Autodesk Inventor part; units mm, degrees
ref_plane "YZ Plane" through (0, 0, 0) normal (1, 0, 0) x (0, 1, 0)
ref_plane "XZ Plane" through (0, 0, 0) normal (0, 1, 0) x (-1, 0, 0)
ref_plane "XY Plane" through (0, 0, 0) normal (0, 0, 1) x (1, 0, 0)
sketch "Sketch1" plane through (0, 0, 0) normal (0, 1, 0) x (-1, 0, 0)
  circle A0 centre (0, 0) radius 4
  arc A1 (-5.0181, 4.8805) -> (5.0181, 4.8805) centre (0, 0) ccw
  arc A2 (9.6094, 20.8964) -> (-9.6094, 20.8964) centre (0, 0) ccw
  arc A3 (-5.0181, 4.8805) -> (-9.6094, 20.8964) centre (-11.9, 11.5737) ccw
  arc A4 (9.6094, 20.8964) -> (5.0181, 4.8805) centre (11.9, 11.5737) ccw
  line L0 (5.0181, 4.8805) -> (-5.0181, 4.8805)
  dimension "d0" = 8
  dimension "d1" = 14
  dimension "d2" = 46
  dimension "d15" = 9.6
  dimension "d17" = 4.6
extrude "Extrusion3" add sketch "Sketch1" along normal blind 1.5
properties part number "crusher_claw"
Model file for the job. Use its own axes, mm. Round coordinates to 2 decimals unless told otherwise and drop trailing zeros. Loops run counter-clockwise (first coordinate to the right, second up) from the corner with the lowest first, then second, coordinate; pieces in that order, holes last. Notation, with made-up numbers: M 73,-37.75 L 100,-37.75 A15 ccw 100,-28.75 Z; hole C 74,65 d11. An arc over 180 degrees is marked long. Put each result on its own line as item: value. Start each with the question number.
Item 1: Mould opens along Z. For faces 1 (the face through (0, 1, 23)), 2 (the face through (0, 0, 8)), 3 (the face through (-2.634, 0.74, 14.083)), 4 (the face through (2.71, 0.74, 14.35)) say: released by +Z, released by -Z, zero draft, split by the parting line, or undercut.
Item 2: Cut at C-C (x = -2.75). List the corners of the cut face in (y, z) (3 decimals), then the cut area to 3 significant figures.
Item 3: Cut at B-B (x = 6.5). List the corners of the cut face in (y, z), then the cut area to 3 significant figures.
Item 4: Cut at D-D (y = 0.25). List the corners of the cut face in (x, z).
Item 5: Drop a flat-ended pin along its axis: P1, Ø6, axis at x = -2, z = 14, coming from the -Y side. Give the stop position or say it passes through.
Item 6: Drill centre lines: line 1 along Z through (x, y) = (0, 0.95); line 2 along X through (y, z) = (1.4, -1.5); line 3 along X through (y, z) = (1.15, -2). Where is each one in solid material? Low to high.
Item 7: Cut at A-A (z = 0). List the corners of the cut face in (x, y), then the cut area to 3 significant figures.
Answer block:
1. face 1: released by +Z
1. face 2: zero draft
1. face 3: undercut
1. face 4: undercut
2. outline: M 0,-6.437 L 1.5,-6.437 L 1.5,-2.905 L 0,-2.905 Z; M 0,2.905 L 1.5,2.905 L 1.5,8.669 L 0,8.669 Z; M 0,14.478 L 1.5,14.478 L 1.5,22.835 L 0,22.835 Z
2. area: 26.5 mm2
3. outline: M 0,-2.6 L 1.5,-2.6 L 1.5,2.6 L 0,2.6 Z; M 0,19.51 L 1.5,19.51 L 1.5,22.06 L 0,22.06 Z
3. area: 11.6 mm2
4. outline: M -9.61,20.9 A9.6 cw -5.02,4.88 A7 ccw long 5.02,4.88 A9.6 cw 9.61,20.9 A23 ccw Z; hole C 0,0 d8
5. P1: y = 0
6. line 1: -7 to -4, 4 to 23
6. line 2: -6.84 to -3.71, 3.71 to 6.84
6. line 3: -6.71 to -3.46, 3.46 to 6.71
7. outline: M -7,0 L -4,0 L -4,1.5 L -7,1.5 Z; M 4,0 L 7,0 L 7,1.5 L 4,1.5 Z
7. area: 9.00 mm2
